Source: CAD feature listing. Evaluate the final solid. Frame: model axes, mm. Coordinates: 2 decimals unless noted, no trailing zeros. Loops run counter-clockwise (first coordinate to the right, second up) from the corner with the lowest first, then second, coordinate; pieces in that order, holes last.
Item 1: Section query A-A, the plane z = 24. Return the cut outline in (x, y), then the cut area to 3 significant figures.
Item 2: Line query: probe 1 along X at (y, z) = (-15.5, 20.5); probe 2 along X at (y, z) = (-37, 36); probe 3 along Y at (x, z) = (110, 20). Output: solid intervals per line, ascending.
Item 3: Pin query (flat end, axial travel): pin 1 Ø4 at (y, z) = (-13.5, 23.5) entering from -X; pin 2 Ø3 at (y, z) = (-1.5, 13.5) entering from +X; pin 3 Ø10 at (x, z) = (53, 5.5) entering from -Y. Return the tip coordinate at first contact, or that it passes through.
```python
from build123d import *

# Parameters (mm, degrees)
BOSS_EXTRUDE1_DEPTH = 40
FILLET1_R           = 2
FILLET2_R           = 2


with BuildPart() as part:
    # Sketch1 → Boss-Extrude1 (new body)
    with BuildSketch(Plane.XY):
        Polygon((0, 0), (2.6534308254274332, -50.694494191060826), (184.70003032872677, -41.165884299703535), (182.04659950329932, 9.528609891357288), align=None)
    extrude(amount=BOSS_EXTRUDE1_DEPTH)

    # Fillet1
    fillet1_edges = [part.edges().sort_by_distance(p)[0] for p in [
        (183.37331491601304, -15.818637204173122, 40),
        (91.02329975164966, 4.764304945678644, 40),
        (183.37331491601304, -15.818637204173122, 0),
        (91.02329975164966, 4.764304945678644, 0),
        (182.04659950329932, 9.528609891357288, 20),
        (184.70003032872677, -41.165884299703535, 20),
    ]]
    fillet(fillet1_edges, radius=FILLET1_R)

    # Fillet2
    # the kernel refuses this fillet: 2 mm, written as the material it takes off along each edge
    with BuildSketch(Plane(origin=(182.59822426289585, -39.27315841843169, 2), x_dir=(0.052270046139774824, -0.9986329867756952, 0), z_dir=(0, 0, -1))) as fillet2_piece_1_section:
        Polygon((0, 0), (FILLET2_R, 0), (FILLET2_R, -FILLET2_R), (-6.3e-16, -FILLET2_R), align=None)
    fillet2_piece_1 = extrude(amount=FILLET2_R, mode=Mode.PRIVATE)
    fillet2_piece_1 = fillet2_piece_1 - Plane(origin=(182.59822426289585, -39.27315841843169, 2), x_dir=(-0.7431006609440385, 0.6691796527873013, 0), z_dir=(0, 0, -1)) * Sphere(FILLET2_R, mode=Mode.PRIVATE)
    add(fillet2_piece_1, mode=Mode.SUBTRACT)
    with BuildSketch(Plane(origin=(4.546156706699275, -48.5926881252299, 2), x_dir=(0, 0, -1), z_dir=(-0.9986329867756953, -0.052270046139774824, 0))) as fillet2_piece_2_section:
        Polygon((0, 0), (FILLET2_R, 0), (FILLET2_R, FILLET2_R), (0, FILLET2_R), align=None)
    fillet2_piece_2 = extrude(amount=FILLET2_R, mode=Mode.PRIVATE)
    fillet2_piece_2 = fillet2_piece_2 - Plane(origin=(4.546156706699275, -48.5926881252299, 2), x_dir=(-0.0369605040783685, 0.7061401568656699, 0.7071067811865475), z_dir=(-0.9986329867756953, -0.052270046139774824, 0)) * Sphere(FILLET2_R, mode=Mode.PRIVATE)
    add(fillet2_piece_2, mode=Mode.SUBTRACT)
    with BuildSketch(Plane(origin=(0.1045400922795495, -1.9972659735513878, 0), x_dir=(-5e-17, 0, 1), z_dir=(0.052270046139774824, -0.9986329867756953, 0))) as fillet2_piece_3:
        with BuildLine():
            CenterArc((FILLET2_R, -FILLET2_R), FILLET2_R, 90, 90.00000000000006)
            Line((-3.3e-16, -FILLET2_R), (0, 0))
            Line((0, 0), (FILLET2_R, 0))
        make_face()
    extrude(amount=46.76388909877601, mode=Mode.SUBTRACT)
    with BuildSketch(Plane(origin=(0.1045400922795495, -1.9972659735513878, 40), x_dir=(-5e-17, 0, -1), z_dir=(0.052270046139774824, -0.9986329867756953, 0))) as fillet2_piece_4:
        with BuildLine():
            CenterArc((FILLET2_R, FILLET2_R), FILLET2_R, 179.99999999999994, 90.00000000000006)
            Line((-1.1e-16, FILLET2_R), (0, 0))
            Line((0, 0), (FILLET2_R, 0))
        make_face()
    extrude(amount=53.763889098776026, mode=Mode.SUBTRACT)
    with BuildSketch(Plane(origin=(0, 0, 1.9999999999999996), x_dir=(0.052270046139775025, -0.9986329867756953, 0), z_dir=(0, 0, 1))) as fillet2_piece_5:
        with BuildLine():
            CenterArc((FILLET2_R, FILLET2_R), FILLET2_R, 180.00000000000034, 89.99999999999966)
            Line((9e-16, FILLET2_R), (0, 0))
            Line((0, 0), (FILLET2_R, 0))
        make_face()
    extrude(amount=36, mode=Mode.SUBTRACT)
    with BuildSketch(Plane(origin=(0.1045400922795352, -1.9972659735513885, 38), x_dir=(-0.05227004613977481, 0.9986329867756952, 0), z_dir=(0, 0, -1))) as fillet2_piece_6:
        with BuildLine():
            CenterArc((2 - FILLET2_R, FILLET2_R), FILLET2_R, 270, 89.99999999999885)
            Line((1.9999999999999998, FILLET2_R), (2, 0))
            Line((2, 0), (2 - FILLET2_R, 1.42e-14))
        make_face()
    revolve(axis=Axis((0.1045400922795352, -1.9972659735513885, 38), (0.9986329867756952, 0.05227004613977481, 0)), revolution_arc=90, mode=Mode.SUBTRACT)
    with BuildSketch(Plane(origin=(0.1045400922795352, -1.9972659735513885, 1.9999999999999996), x_dir=(-0.05227004613977481, 0.9986329867756952, 0), z_dir=(1e-17, -1.1e-16, 1))) as fillet2_piece_7:
        with BuildLine():
            CenterArc((2 - FILLET2_R, -FILLET2_R), FILLET2_R, 1.15136e-12, 89.99999999999886)
            Line((1.9999999999999998, -FILLET2_R), (2, 0))
            Line((2, 0), (2 - FILLET2_R, -1.42e-14))
        make_face()
    revolve(axis=Axis((0.1045400922795352, -1.9972659735513885, 1.9999999999999996), (-0.9986329867756952, -0.05227004613977481, 0)), revolution_arc=90, mode=Mode.SUBTRACT)
    with BuildSketch(Plane(origin=(4.650696798978822, -50.58995409878128, 0), x_dir=(-0.05227004613977483, 0.9986329867756953, 0), z_dir=(0.9986329867756952, 0.052270046139774824, 0))) as fillet2_piece_8:
        with BuildLine():
            CenterArc((FILLET2_R, FILLET2_R), FILLET2_R, 180, 90)
            Line((-5e-17, FILLET2_R), (0, 0))
            Line((0, 0), (FILLET2_R, 0))
        make_face()
    extrude(amount=178.29580027300779, mode=Mode.SUBTRACT)
    with BuildSketch(Plane(origin=(2.6534308254274332, -50.694494191060826, 2), x_dir=(-0.05227004613977479, 0.9986329867756952, 0), z_dir=(0, 0, 1))) as fillet2_piece_9:
        with BuildLine():
            CenterArc((FILLET2_R, -FILLET2_R), FILLET2_R, 90, 90)
            Line((-1.444e-14, -FILLET2_R), (0, 0))
            Line((0, 0), (FILLET2_R, 0))
        make_face()
    extrude(amount=43, mode=Mode.SUBTRACT)


solid = part.part
```
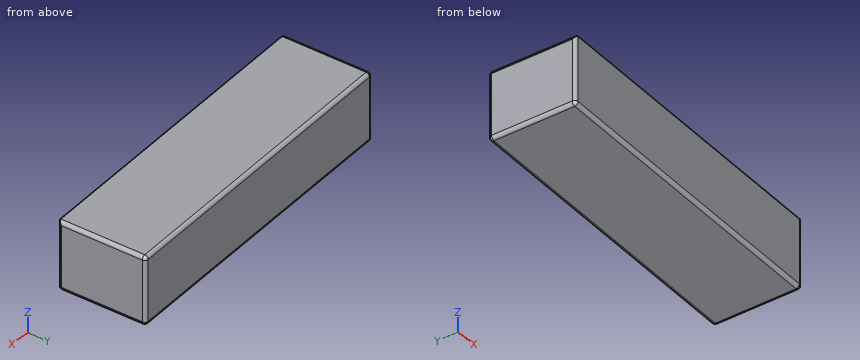
Verdict:
1. outline: (0.1, -2) - (2.55, -48.7) arc R2 ccw to (4.65, -50.59) - (182.7, -41.27) arc R2 ccw to (184.6, -39.17) - (182.15, 7.53) arc R2 ccw to (180.05, 9.42) - (2, 0.1) arc R2 ccw to start
1. area: 9,250 mm2
2. probe 1: x = 0.81 to 183.36
2. probe 2: x = 1.94 to 184.48
2. probe 3: y = -45.08 to 5.76
3. pin 1: stops at x = 0.6
3. pin 2: stops at x = 182.7
3. pin 3: stops at y = -48.32
